Source: CAD feature listing. Evaluate the final solid. Frame: model axes, mm. Face numbers are marked on the shaded views. Give positions to 0.01 mm unless a question says otherwise; leave off trailing zeros. Order: outer loops, then holes, each group sorted by start corner. A loop starts at its lowest first (then second) coordinate and runs counter-clockwise, first axis right, second up.
1) First-contact query: P1, Ø1, axis at y = -7.5, z = 3.5, coming from the +X side; P2, Ø1, axis at y = 12, z = 4, coming from the -X side; P3, Ø1.5, axis at x = -1.5, z = 1.5, coming from the -Y side. Flat tips, straight axial feed; report the tip coordinate or a pass-through.
2) Section C-C, the plane z = 1.6. Return loops of the section in (x, y), plus the area to 3 significant figures.
3) Material intervals for line 1 (Y direction, x = 0, z = 2.9); line 2 (X direction, y = 3, z = 2.6); line 3 (Y direction, x = 50, z = 3.9), sorted ascending.
4) Section A-A, the plane x = 0. Return loops of the section in (y, z), plus the area to 3 significant figures.
5) Section B-B, the plane y = 0. Return loops of the section in (x, z).
6) Section D-D, the plane y = -14. Return loops of the section in (x, z), plus the area to 3 significant figures.
7) Draft query along X for the marked faces 1, 2 and 3. Return one class per face: released by +X, released by -X, zero draft, split by the parting line, or undercut.
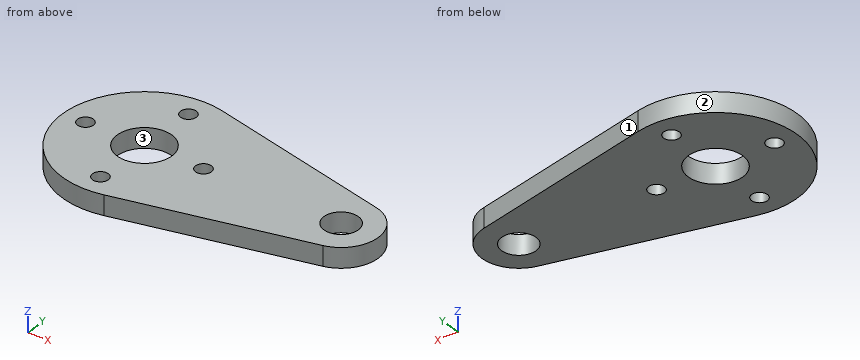
```python
from build123d import *

# Parameters (mm, degrees)
SKETCH1_R           = 6.9
SKETCH1_R_2         = 4.35
SKETCH1_R_3         = 2
BOSS_EXTRUDE1_DEPTH = 5


with BuildPart() as part:
    # Sketch1 → Boss-Extrude1 (new body)
    with BuildSketch(Plane.XY):
        with BuildLine():
            Line((4.6989, 20.159621494), (52.12245, 9.105915989))
            ThreePointArc((52.12245, 9.105915989), (59.35, 0), (52.12245, -9.105915989))
            Line((52.12245, -9.105915989), (4.6989, -20.159621494))
            ThreePointArc((4.6989, -20.159621494), (-20.7, 0), (4.6989, 20.159621494))
        make_face()
        Circle(SKETCH1_R, mode=Mode.SUBTRACT)
        with Locations((50, 0)):
            Circle(SKETCH1_R_2, mode=Mode.SUBTRACT)
        with Locations((15, 0)):
            Circle(SKETCH1_R_3, mode=Mode.SUBTRACT)
        with Locations((0, -15)):
            Circle(SKETCH1_R_3, mode=Mode.SUBTRACT)
        with Locations((-15, 0)):
            Circle(SKETCH1_R_3, mode=Mode.SUBTRACT)
        with Locations((0, 15)):
            Circle(SKETCH1_R_3, mode=Mode.SUBTRACT)
    extrude(amount=BOSS_EXTRUDE1_DEPTH)


solid = part.part
```
From the geometry:
1. P1: stops at x = 56.2
1. P2: stops at x = -17.21
1. P3: stops at y = -20.69
2. outline: (4.7, -20.16) - (52.12, -9.11) arc R9.35 ccw to (52.12, 9.11) - (4.7, 20.16) arc R20.7 ccw (long way) to start; hole circle Ø4 at (-15, 0); hole circle Ø13.8 at (0, 0); hole circle Ø4 at (0, -15); hole circle Ø4 at (0, 15); hole circle Ø4 at (15, 0); hole circle Ø8.7 at (50, 0)
2. area: 2,090 mm2
3. line 1: y = -20.7 to -17, -13 to -6.9, 6.9 to 13, 17 to 20.7
3. line 2: x = -20.48 to -6.21, 6.21 to 46.85, 53.15 to 58.86
3. line 3: y = -9.6 to -4.35, 4.35 to 9.6
4. outline: (-20.7, 0) - (-17, 0) - (-17, 5) - (-20.7, 5) - close; (-13, 0) - (-6.9, 0) - (-6.9, 5) - (-13, 5) - close; (6.9, 0) - (13, 0) - (13, 5) - (6.9, 5) - close; (17, 0) - (20.7, 0) - (20.7, 5) - (17, 5) - close
4. area: 98.0 mm2
5. outline: (-20.7, 0) - (-17, 0) - (-17, 5) - (-20.7, 5) - close; (-13, 0) - (-6.9, 0) - (-6.9, 5) - (-13, 5) - close; (6.9, 0) - (13, 0) - (13, 5) - (6.9, 5) - close; (17, 0) - (45.65, 0) - (45.65, 5) - (17, 5) - close; (54.35, 0) - (59.35, 0) - (59.35, 5) - (54.35, 5) - close
6. outline: (-15.25, 0) - (-1.73, 0) - (-1.73, 5) - (-15.25, 5) - close; (1.73, 0) - (31.13, 0) - (31.13, 5) - (1.73, 5) - close
6. area: 215 mm2
7. face 1: released by +X
7. face 2: split by the parting line
7. face 3: undercut
